from build123d import *


with BuildPart() as f1:
    # F0 (on Front) → F1 (revolve)
    with BuildSketch(Plane.XZ):
        with BuildLine():
            Line((13.4330698064, -46.3841338361), (15.2060489871, -46.3841338361))
            Line((15.2060489871, -46.3841338361), (15.2060312931, -43.6701662838))
            Line((15.2060312931, -43.6701662838), (14.2253357917, -43.6701662838))
            Line((14.2253357917, -43.6701662838), (14.2253357917, -41.9087485828))
            Line((14.2253357917, -41.9087485828), (15.2060145196, -41.0973673151))
            Line((15.2060145196, -41.0973673151), (15.2057230017, 3.6168700514))
            Line((15.2057230017, 3.6168700514), (15.2057230017, 5.1168700514))
            Line((15.2057230017, 5.1168700514), (14.7057230017, 5.1168700514))
            add(Edge.make_bspline(
                [(14.7057230017, 5.1168700514), (13.6535132095, 21.3489830368), (10.0671686232, 33.6324311793), (0, 33.2716815174)],
                knots=[0, 0, 0, 0, 31.7640000266, 31.7640000266, 31.7640000266, 31.7640000266], degree=3))
            Line((0, 33.2716815174), (0.2071067812, -45.3841338361))
            Line((0.2071067812, -45.3841338361), (1.2071067812, -46.3841338361))
            Line((1.2071067812, -46.3841338361), (7.4330698064, -46.3841338361))
            Line((7.4330698064, -46.3841338361), (8.4330698064, -46.3841338361))
            Line((8.4330698064, -46.3841338361), (9.4330698064, -45.3841338361))
            Line((9.4330698064, -45.3841338361), (10.4330698064, -45.3841338361))
            Line((10.4330698064, -45.3841338361), (11.4330698064, -46.3841338361))
            Line((11.4330698064, -46.3841338361), (13.4330698064, -46.3841338361))
        make_face()
    revolve(axis=Axis((0.1035533906, 0, -6.0562261594), (0.0026330674, 0, -0.9999965335)))


solid = f1.part
Build history of the part. All positions in model axes, mm. Give positions to 0.01 mm unless a question says otherwise; leave off trailing zeros. Use one line per item in the form item = value. Start each with the question number.
1. Drop flat-ended pins along their axis: pin 1 Ø4 at (y, z) = (-7, -28) entering from -X; pin 2 Ø10 at (x, y) = (4.5, -7) entering from -Z; pin 3 Ø12 at (y, z) = (-7, -8) entering from +X. Give the stop position or say it passes through.
2. Probe line 1 (Z direction, x = -2.5, y = 14.5); line 2 (Y direction, x = 12.5, z = -17); line 3 (Y direction, x = 4.5, z = -18). List the from-to ranges inside material, lowest first. Write a range as [from, to].
3. Two-plate mould, pull along Z, no slides. Class faces 1 (the face through (13.58, -4.21, -42.78)), 2 (the face through (-0.1, 1.41, -46.39)): released by +Z, released by -Z, zero draft, split by the parting line, or undercut.
Conclusion:
q1.pin_1 = -14.03
q1.pin_2 = -46.41
q1.pin_3 = 15.17
q2.line_1 = [-46.43, -43.72], [-41.36, 5.07]
q2.line_2 = [-8.62, 8.62]
q2.line_3 = [-14.42, 14.42]
q3.face_1 = undercut
q3.face_2 = released by -Z
